Check sheet for the modelled part. Datum: model origin and axes. Units: mm. Face numbers are marked on the shaded views. A direction names the side the tool comes from. Give positions to 0.01 mm unless a question says otherwise; leave off trailing zeros. Loops run counter-clockwise (first coordinate to the right, second up) from the corner with the lowest first, then second, coordinate; pieces in that order, holes last. Notation, with made-up numbers: (14, -27.75) -> (60, -27.75) arc R19 cw to (60, -6.75) -> close; hole circle Ø2 at (81, 83.5). An arc over 180 degrees is marked (long way). Write each question's results on one line, items separated by ' | '. Start each with the question number.
1. Gauge pin test, flat ends, axial feed: pin 1 Ø6 at (y, z) = (-8, 3.5) entering from +X; pin 2 Ø2.5 at (y, z) = (-25.5, 8.5) entering from +X (3 decimals); pin 3 Ø6 at (x, z) = (25, 8) entering from +Y. Record the tip position at first contact, or that the pin passes through.
2. Cross-section at C-C on z = 5.5. Record the boundary of the cut face in (x, y) (1 decimal), and give its area (3 significant figures).
3. Mould release check, pull along Y, two halves, no side actions. Record for the marked faces 1, 2, 3 and 4: +Y half, -Y half, draft (parallel to the pull), parting line (faces both ways), or undercut.
4. Material ranges on L1, parallel to Z at x = 30, y = -20 (3 decimals); L2, parallel to X at y = -22, z = 11.75 (3 decimals); L3, parallel to X at y = -21, z = 10.25 (3 decimals), recorded low to high. Write a range as from..to.
5. Cross-section at B-B on z = 2.5. Record the boundary of the cut face in (x, y) (1 decimal), and give its area (3 significant figures).
6. Cross-section at A-A on x = 23. Record the boundary of the cut face in (y, z) (3 decimals).
7. Cross-section at D-D on y = -7.5. Record the boundary of the cut face in (x, z) (3 decimals), and give its area (3 significant figures).
8. Tool access check on the marked faces 5, 6 and 7. Record the directions out of +Z, -Z, +X, -X, +Y, -Y that give a thin tool (end or side, any length) a straight path to the whole face; none if there is none.
Autodesk Inventor part; units mm, degrees
ref_plane "YZ Plane" through (0, 0, 0) normal (1, 0, 0) x (0, 1, 0)
ref_plane "XZ Plane" through (0, 0, 0) normal (0, 1, 0) x (-1, 0, 0)
ref_plane "XY Plane" through (0, 0, 0) normal (0, 0, 1) x (1, 0, 0)
sketch "Sketch2" plane through (0, 0, 0) normal (0, 0, 1) x (1, 0, 0)
  line L0 (0, 0) -> (51.3842, 0)
  line L1 (51.3842, 0) -> (65.3796, -24.2407)
  line L2 (65.3796, -24.2407) -> (61.3791, -31.1698)
  line L3 (65.3796, -24.2407) -> (73.3806, -24.2407) construction
  line L4 (61.3791, -31.1698) -> (19.4691, -31.1698)
  line L5 (19.4691, -31.1698) -> (24.9555, -21.6671)
  line L6 (19.4691, -31.1698) -> (30.4419, -31.1698) construction
  line L7 (24.9555, -21.6671) -> (0, 0)
  line L8 (51.3842, 0) -> (58.6918, 0) construction
  line L9 (48.8733, -7.5723) -> (70.4506, -7.5723) construction
  circle A0 centre (48.2959, -6.6229) radius 2.2225
  circle A1 centre (59.662, -26.2588) radius 2.2225
  dimension "d0" = 51.3842
  dimension "d1" = 27.9908
  dimension "d2" = 120
  dimension "d3" = 8.001
  dimension "d4" = 120
  dimension "d5" = 41.91
  dimension "d6" = 10.9728
  dimension "d7" = 60
  dimension "d15" = 4.445
  dimension "d16" = 4.445
extrude "Extrusion1" add sketch "Sketch2" along normal blind 15.24
sketch "Sketch3" plane through (65.3796, -24.2407, 15.24) normal (0.866, -0.5, 0) x (0, 0, -1)
  point P0 (15.24, -11.6967)
sketch "Sketch4" plane through (65.3796, -24.2407, 15.24) normal (0.866, -0.5, 0) x (0, 0, -1)
  line L0 (15.24, -8.001) -> (0, -8.001)
  line L1 (0, -8.001) -> (3.175, -8.001)
  line L2 (15.24, 0) -> (0, 0)
  line L3 (3.175, -8.001) -> (12.065, -8.001)
  line L4 (12.065, -8.001) -> (12.065, 0)
  line L5 (12.065, 0) -> (3.175, 0)
  line L6 (3.175, 0) -> (3.175, -8.001)
  point P0 (15.24, -11.6967)
  point P1 (3.175, 0)
  point P2 (12.065, -8.001)
  dimension "d19" = 3.175
  dimension "d20" = 8.89
sketch "Sketch5" plane through (19.4691, -31.1698, 0) normal (0, -1, 0) x (1, 0, 0)
  point P0 (-19.4691, 0)
extrude "Extrusion2" cut sketch "Sketch4" against normal blind 127
sketch "Sketch6" plane through (19.4691, -31.1698, 0) normal (0, -1, 0) x (1, 0, 0)
  point P0 (-19.4691, 0)
sketch "Sketch7" plane through (19.4691, -31.1698, 0) normal (0, -1, 0) x (1, 0, 0)
  line L0 (0, 0) -> (41.91, 0)
  line L1 (41.91, 3.175) -> (41.91, 12.065)
  line L2 (41.91, 0) -> (41.91, 3.175)
  line L3 (41.91, 12.065) -> (-12.0777, 12.065)
  line L4 (41.91, 3.175) -> (5.08, 3.175)
  line L5 (5.08, 12.065) -> (41.91, 12.065)
  line L6 (41.91, 12.065) -> (41.91, 3.175)
  line L7 (6.7536, 12.065) -> (6.7536, 3.175)
  line L8 (41.91, 3.175) -> (-12.0777, 3.175)
  point P0 (-19.4691, 0)
  dimension "d23" = 36.83
extrude "Extrusion3" [suppressed]
sketch "Sketch8" plane through (0, 0, 0) normal (0, 1, 0) x (1, 0, 0)
  line L0 (65.3796, -3.175) -> (23.3934, -3.175)
  line L1 (24.5491, -3.175) -> (23.3934, -3.175)
  line L2 (23.3934, -12.065) -> (7.3914, -12.065)
  line L3 (24.5491, -3.175) -> (23.3934, -3.175)
  line L4 (23.3934, -3.175) -> (23.3934, -12.065)
  line L5 (23.3934, -12.065) -> (24.5491, -12.065)
  line L6 (24.5491, -12.065) -> (24.5491, -3.175)
  point P0 (0, 0)
extrude "Extrusion4" cut sketch "Sketch8" along normal mid plane 15.24
sketch "Sketch9" plane through (61.3791, -21.9311, 3.175) normal (-1, 0, 0) x (0, 0, 1)
  point P0 (-3.175, 21.9311)
sketch "Sketch10" plane through (65.3796, -24.2407, 12.065) normal (0.866, 0.5, 0) x (0, 0, -1)
  line L0 (8.89, 0) -> (0, 0)
  line L1 (8.89, 4.0005) -> (8.89, 8.001)
  line L2 (0, 0) -> (8.89, 0)
  line L3 (8.89, 0) -> (8.89, 8.001)
  line L4 (8.89, 8.001) -> (0, 8.001)
  line L5 (0, 8.001) -> (0, 0)
  point P0 (12.065, 53.6829)
extrude "Extrusion5" cut sketch "Sketch10" against normal blind 15.24
sketch "Sketch11" plane through (19.4691, -31.1698, 0) normal (0, -1, 0) x (1, 0, 0)
  line L0 (42.4154, 3.175) -> (37.9704, 3.175)
  line L1 (42.4154, 3.175) -> (6.2959, 3.175)
  line L2 (6.2959, 3.175) -> (6.2959, 12.065)
  line L3 (6.2959, 12.065) -> (42.4154, 12.065)
  line L4 (42.4154, 12.065) -> (42.4154, 3.175)
  point P0 (-19.4691, 0)
extrude "Extrusion6" cut sketch "Sketch11" against normal blind 127
sketch "Sketch12" plane through (24.5491, 0, 3.175) normal (-1, 0, 0) x (0, 0, 1)
  point P0 (-3.175, 0)
sketch "Sketch13" plane through (0, 0, 0) normal (0, 1, 0) x (1, 0, 0)
  line L0 (25.765, -3.175) -> (24.5491, -3.175)
  line L1 (25.765, -3.175) -> (25.765, -12.065)
  line L2 (24.5491, -3.175) -> (25.765, -3.175)
  line L3 (25.765, -3.175) -> (25.765, -12.065)
  line L4 (25.765, -12.065) -> (24.5491, -12.065)
  line L5 (24.5491, -12.065) -> (24.5491, -3.175)
  point P0 (0, 0)
extrude "Extrusion7" cut sketch "Sketch13" against normal blind 2.54
chamfer "Chamfer1" distance 0.635 angle 45 6 edges at (61.3791, -31.1698, 13.6525) (65.3796, -24.2407, 13.6525) (65.3796, -24.2407, 1.5875) (61.3791, -31.1698, 1.5875) (51.3842, 0, 13.6525) (51.3842, 0, 1.5875)
properties part number "Non Colour Claw" material "Iron, Gray"
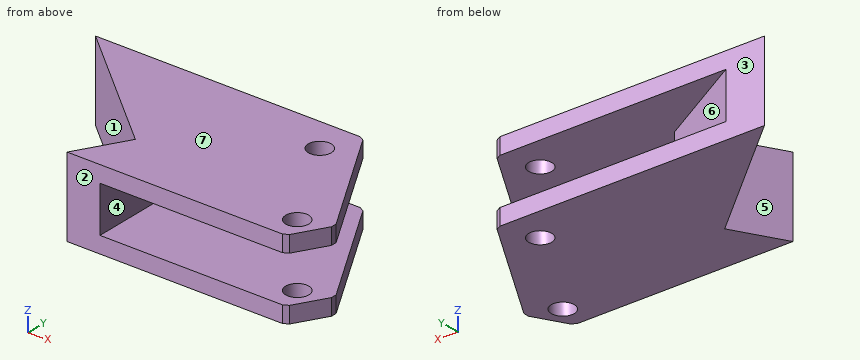
Geometry says:
1) pin 1: x = 57.72 | pin 2: x = 25.765 | pin 3: y = -8.43
2) outline: (0, 0) -> (25, -21.7) -> (19.5, -31.2) -> (25.8, -31.2) -> (25.8, -10.6) -> (7.4, 0) -> close | area: 224 mm^2
3) face 1: undercut | face 2: -Y half | face 3: +Y half | face 4: draft
4) L1: 0..3.175, 12.065..15.24 | L2: 24.763..25.765 | L3: 24.187..25.765
5) outline: (0, 0) -> (25, -21.7) -> (19.5, -31.2) -> (60.7, -31.2) -> (61.7, -30.6) -> (65.1, -24.8) -> (65.1, -23.7) -> (51.7, -0.5) -> (50.7, 0) -> close; hole circle Ø4.4 at (48.3, -6.6); hole circle Ø4.4 at (59.7, -26.3) | area: 1,340 mm^2
6) outline: (-31.17, 0) -> (-25.054, 0) -> (-25.054, 15.24) -> (-31.17, 15.24) -> close; (-19.969, 0) -> (0, 0) -> (0, 3.175) -> (-9.012, 3.175) -> (-9.012, 12.065) -> (0, 12.065) -> (0, 15.24) -> (-19.969, 15.24) -> close
7) outline: (8.638, 0) -> (46.254, 0) -> (46.254, 3.175) -> (20.382, 3.175) -> (20.382, 12.065) -> (46.254, 12.065) -> (46.254, 15.24) -> (8.638, 15.24) -> close; (50.338, 0) -> (55.714, 0) -> (55.714, 3.175) -> (50.338, 3.175) -> close; (50.338, 12.065) -> (55.714, 12.065) -> (55.714, 15.24) -> (50.338, 15.24) -> close | area: 377 mm^2
8) face 5: +Z, -Z, -X | face 6: +X, +Y | face 7: +Z, +X, -X, +Y, -Y
